Read the model definition and answer for the solid it produces. Units are mm, in the model's axes. Face numbers are marked on the shaded views. Coordinates: 2 decimals unless noted, no trailing zeros. Write each loop counter-clockwise with the first axis right and the second up, starting at its lowest first coordinate (ties: lowest second). Pieces come first, ordered by that corner, then holes. Notation, with made-up numbers: (69.25, 80) -> (127.25, 80) arc R15 cw to (127.25, 92) -> close; hole circle Ø10 at (77.25, 43). An arc over 180 degrees is marked (long way). Answer as a JSON object with one key per item and string values. Group by question number.
(1) Straight lines are drawn through the part: L1, parallel to X at y = 0.5, z = 0.25; L2, parallel to X at y = -7, z = 0; L3, parallel to Y at x = -10.5, z = 0.75. For each, find the intervals that lie inside material, in ascending order.
(2) Find section D-D (x = -12). Give the vertices of the cut face in (y, z).
(3) Find section B-B (z = 0.5). Give the vertices of the cut face in (x, y) (1 decimal).
(4) Flat-ended cylindrical pins translate along their axes: P1, Ø4, axis at y = -14.5, z = -2.5, coming from the -X side; P2, Ø2, axis at y = -18, z = 2, coming from the -X side; P3, Ø1.5, axis at x = -11.5, z = -2, coming from the +Y side. Find the tip coordinate at first contact, or state that the pin passes through.
(5) For a pull along X with two mould halves and no side action, classify the marked faces 1, 2 and 3 as +X half, -X half, draft (parallel to the pull), parting line (faces both ways), or undercut.
(6) Find section C-C (y = -19.75). Give the vertices of the cut face in (x, z).
(7) Find section A-A (x = 0). Give the vertices of the cut face in (y, z), then the cut area to 3 significant figures.
from build123d import *

# Parameters (mm, degrees)
SKETCH2_R           = 19.05
BOSS_EXTRUDE1_DEPTH = 44.45
SCALE1_SCALE        = 0.083333333


with BuildPart() as part:
    # Sketch2 → Boss-Extrude1 (new body, symmetric)
    with BuildSketch(Plane.XY):
        with BuildLine():
            Line((-246.541287735, -61.175642711), (-59.652807836, -4.602086269))
            ThreePointArc((-59.652807836, -4.602086269), (-48.980567788, 1.8190908), (-42.643954444, 12.541756231))
            ThreePointArc((-42.643954444, 12.541756231), (0, 44.45), (42.643954444, 12.541756231))
            ThreePointArc((42.643954444, 12.541756231), (48.980567788, 1.8190908), (59.652807836, -4.602086269))
            Line((59.652807836, -4.602086269), (246.541287735, -61.175642711))
            ThreePointArc((246.541287735, -61.175642711), (261.864746274, -74.055516083), (263.100383875, -94.034823363))
            ThreePointArc((263.100383875, -94.034823363), (0, -279.4), (-263.100383875, -94.034823363))
            ThreePointArc((-263.100383875, -94.034823363), (-261.864746274, -74.055516083), (-246.541287735, -61.175642711))
        make_face()
        Circle(SKETCH2_R, mode=Mode.SUBTRACT)
    extrude(amount=BOSS_EXTRUDE1_DEPTH, both=True)


with BuildPart() as part_1:
    # Scale1: scaled about (0, 0, 0)
    add(part.part.scale(SCALE1_SCALE))


solid = part_1.part
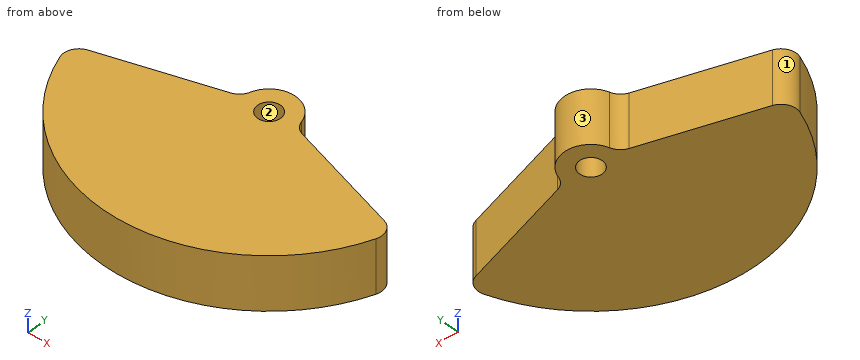
Results below:
{
 "1": {"L1": "x = -3.8 to -1.51, 1.51 to 3.8", "L2": "x = -22.04 to 22.04", "L3": "y = -20.78 to -2.06"},
 "2": {"outline": "(-19.95, -3.7) -> (-2.51, -3.7) -> (-2.51, 3.7) -> (-19.95, 3.7) -> close"},
 "3": {"outline": "(-21.9, -7.8) arc R23.3 ccw to (21.9, -7.8) arc R2.1 ccw to (20.5, -5.1) -> (5, -0.4) arc R2.1 cw to (3.6, 1) arc R3.7 ccw to (-3.6, 1) arc R2.1 cw to (-5, -0.4) -> (-20.5, -5.1) arc R2.1 ccw to start; hole circle Ø3.2 at (0, 0)"},
 "4": {"P1": "stops at x = -19.64", "P2": "stops at x = -15.91", "P3": "stops at y = -2.13"},
 "5": {"face 1": "-X half", "face 2": "undercut", "face 3": "parting line"},
 "6": {"outline": "(-12.33, -3.7) -> (12.33, -3.7) -> (12.33, 3.7) -> (-12.33, 3.7) -> close"},
 "7": {"outline": "(-23.28, -3.7) -> (-1.59, -3.7) -> (-1.59, 3.7) -> (-23.28, 3.7) -> close; (1.59, -3.7) -> (3.7, -3.7) -> (3.7, 3.7) -> (1.59, 3.7) -> close", "area": "176 mm2"}
}
